Can you work these out from the model? Positions are in its coordinate system, mm. A direction names the side the tool comes from. Give positions to 0.01 mm unless a question says otherwise; leave off trailing zeros. Write each loop counter-clockwise with the first axis right and the second up, starting at its lowest first coordinate (ties: lowest second). Pieces come first, ordered by that corner, then holes.
from build123d import *

# Parameters (mm, degrees)
F1_DEPTH = 762
F3_DEPTH = 254
F4_DEPTH = 1143


with BuildPart() as f1:
    # F0 (on Front) → F1 (new body)
    with BuildSketch(Plane.XZ):
        Polygon((254, 254), (0, 0), (2032, 0), (1778, 254), (1524, 254), (1524, 1016), (508, 1016), (508, 254), align=None)
    extrude(amount=F1_DEPTH)

    # F2 (on face) → F3 (join)
    with BuildSketch(Plane.XZ.offset(762)):
        with BuildLine():
            Line((762, 1016), (508, 1016))
            ThreePointArc((508, 1016), (1016, 508), (1524, 1016))
            Line((1524, 1016), (1270, 1016))
            ThreePointArc((1270, 1016), (1016, 762.9418953538), (762, 1016))
        make_face()
    extrude(amount=F3_DEPTH)

    # F4 (cut): a face of the model
    f4_faces = [f1.faces().sort_by_distance(p)[0] for p in [
        (1016, -762, 908.631847947),
    ]]
    extrude(f4_faces, amount=-F4_DEPTH, mode=Mode.SUBTRACT)


solid = f1.part
(1) Imagine slicing it at B-B, the plane x = 1016. Write out the boundary of the cut face in (y, z).
Returned:
outline: (-1016, 508) - (-762, 508) - (-762, 0) - (0, 0) - (0, 762.94) - (-1016, 762.94) - close
(2) Will these pins go through, and if not, where does the flat tip stop? P1, Ø10, axis at y = -267, z = 197.5, coming from the -X side; P2, Ø8, axis at x = 1423.5, z = 248.5, coming from the -Y side; P3, Ø4, axis at y = -896.5, z = 569, coming from the +X side.
Returned:
P1: stops at x = 192.5
P2: stops at y = -762
P3: stops at x = 1261.03
(3) If I drill on L1, parallel to Y at x = 454, z = 57; L2, parallel to Z at x = 492.5, y = -447; L3, parallel to X at y = -310, z = 342, over which ranges is the centre line in solid material (lowest first)?
Returned:
L1: y = -762 to 0
L2: z = 0 to 254
L3: x = 508 to 1524
(4) For faces 4 (the face through (1399, -501, 1016)), 5 (the face through (1009, -1016, 709)), 6 (the face through (1653, -376, 254)), 7 (the face through (1004.829, -887.222, 508.123)), 8 (the face through (383, -376, 254)), which set-ups out of +Z, -Z, +X, -X, +Y, -Y let a thin tool reach every point of the face, with its end or its side?
Returned:
face 4: +Z, +X, -X, +Y, -Y
face 5: +Z, -Z, +X, -X, -Y
face 6: +Z, +X, +Y, -Y
face 7: -Z, -Y
face 8: +Z, -X, +Y, -Y
(5) Imagine slicing it at A-A, the plane z = 897. Write out the boundary of the cut face in (x, y).
Returned:
outline: (508, -762) - (522.13, -762) - (522.13, -1016) - (792.1, -1016) - (792.1, 0) - (508, 0) - close; (1239.9, -1016) - (1509.87, -1016) - (1509.87, -762) - (1524, -762) - (1524, 0) - (1239.9, 0) - close
(6) Imagine slicing it at C-C, the plane y = -64. Write out the boundary of the cut face in (x, z).
Returned:
outline: (0, 0) - (2032, 0) - (1778, 254) - (1524, 254) - (1524, 1016) - (1270, 1016) arc R254 cw to (762, 1016) - (508, 1016) - (508, 254) - (254, 254) - close
(7) Imagine slicing it at D-D, the plane z = 390.5. Write out the boundary of the cut face in (x, y).
Returned:
outline: (508, -762) - (1524, -762) - (1524, 0) - (508, 0) - close
(8) If we mould it in two halves opening along X, with no side actions, what happens to faces 1 (the face through (1021.572, -515.112, 763.003)), 2 (the face through (508, -376, 640)), 3 (the face through (637, -501, 1016))? For each: +X half, -X half, draft (parallel to the pull), parting line (faces both ways), or undercut.
Returned:
face 1: undercut
face 2: -X half
face 3: draft
